```python
from build123d import *

# Parameters (mm, degrees)
SKETCH1_W            = 40
SKETCH1_H            = 40
BOSS_EXTRUDE1_DEPTH  = 650
BOSS_EXTRUDE2_START  = 550
SKETCH3_R            = 9.5
BOSS_EXTRUDE2_DEPTH  = 200
SKETCH8_R            = 150
BOSS_EXTRUDE3_DEPTH  = 10
SKETCH9_W            = 105
SKETCH9_H            = 8
SKETCH9_H_2          = 40
BOSS_EXTRUDE4_DEPTH  = 40
FILLET1_R            = 10
SKETCH10_R           = 6
CUT_EXTRUDE1_DEPTH   = 735.31209305
CUT_EXTRUDE2_DEPTH   = 767.485485838
CUT_EXTRUDE5_DEPTH   = 767.485485838
SHELL2_START         = -18
SHELL2_DEPTH         = 36
SHELL2_START_2       = 22
SHELL2_2_DEPTH       = 6
SHELL2_START_3       = 8.0000001
SHELL2_3_DEPTH       = 13.9999999
SHELL2_START_4       = -10
SHELL2_4_DEPTH       = 1.9999999
SHELL2_START_5       = -552
SHELL2_5_OUTLINE_W   = 36
SHELL2_5_OUTLINE_H   = 8
SHELL2_5_OUTLINE_H_2 = 16.0000002
SHELL2_5_DEPTH       = 1300
SHELL2_6_OUTLINE_W   = 105
SHELL2_6_OUTLINE_H   = 8
SHELL2_6_OUTLINE_H_2 = 16.0000002
SHELL2_6_DEPTH       = 36
SHELL2_START_6       = -748
SHELL2_7_OUTLINE_R   = 7.5
SHELL2_7_DEPTH       = 196
SHELL2_START_7       = 552
SHELL2_8_DEPTH       = 196
SHELL2_START_8       = -66
SHELL2_9_DEPTH       = 4
SHELL2_START_9       = 62
SHELL2_10_DEPTH      = 4
SKETCH12_R           = 12.5
CUT_EXTRUDE3_DEPTH   = 70
SKETCH13_W           = 30
SKETCH13_H           = 30
CUT_EXTRUDE4_DEPTH   = 20


with BuildPart() as part:
    # Sketch1 → Boss-Extrude1 (new, symmetric)
    with BuildSketch(Plane.XY):
        Rectangle(SKETCH1_W, SKETCH1_H)
    extrude(amount=BOSS_EXTRUDE1_DEPTH, both=True)

    # Sketch3 → Boss-Extrude2 (add)
    with BuildSketch(Plane.XY.offset(BOSS_EXTRUDE2_START)):
        with Locations(Location((0, 25, 0), (0, 0, 211.756863859))):
            Circle(SKETCH3_R)
    boss_extrude2 = extrude(amount=BOSS_EXTRUDE2_DEPTH)

    # Sketch8 → Boss-Extrude3 (add)
    with BuildSketch(Plane(origin=(0, 20, 0), x_dir=(1, 0, 0), z_dir=(0, 1, 0))):
        with Locations(Location((0, 0, 0), (0, 0, 277.662255661))):
            Circle(SKETCH8_R)
    extrude(amount=BOSS_EXTRUDE3_DEPTH)

    # Sketch9 → Boss-Extrude4 (add)
    with BuildSketch(Plane.XZ.offset(-20)):
        with Locations((72.5, -64)):
            Rectangle(SKETCH9_W, SKETCH9_H)
        with Locations((72.5, 64)):
            Rectangle(SKETCH9_W, SKETCH9_H)
        with Locations((-72.5, 0)):
            Rectangle(SKETCH9_W, SKETCH9_H_2)
    extrude(amount=BOSS_EXTRUDE4_DEPTH)

    # Fillet1
    fillet1_edges = [part.edges().sort_by_distance(p)[0] for p in [
        (125, -20, -64),
        (125, -20, 64),
    ]]
    fillet(fillet1_edges, radius=FILLET1_R)

    # Sketch10 → Cut-Extrude1 (cut, through all)
    with BuildSketch(Plane.XY.offset(68)):
        with Locations((105, 0)):
            Circle(SKETCH10_R)
    extrude(amount=-CUT_EXTRUDE1_DEPTH, mode=Mode.SUBTRACT)

    # Sketch11 → Cut-Extrude2 (cut, through all)
    with BuildSketch(Plane(origin=(0, 30, 0), x_dir=(1, 0, 0), z_dir=(0, 1, 0))):
        with BuildLine():
            Line((105, 17.5), (150, 17.5))
            Line((150, 17.5), (150, -17.5))
            Line((150, -17.5), (105, -17.5))
            ThreePointArc((105, -17.5), (87.5, 0), (105, 17.5))
        make_face()
    extrude(amount=-CUT_EXTRUDE2_DEPTH, mode=Mode.SUBTRACT)

    # Mirror1: Boss-Extrude2 across plane
    add(boss_extrude2.mirror(Plane.XY))

    # Sketch14 → Cut-Extrude5 (cut, through all)
    with BuildSketch(Plane(origin=(0, 30, 0), x_dir=(1, 0, 0), z_dir=(0, 1, 0))):
        with BuildLine():
            Line((-106.066017178, 106.066017178), (-98.994949366, 98.994949366))
            ThreePointArc((-98.994949366, 98.994949366), (-140, 0), (-98.994949366, -98.994949366))
            Line((-98.994949366, -98.994949366), (-106.066017178, -106.066017178))
            ThreePointArc((-106.066017178, -106.066017178), (-150, 0), (-106.066017178, 106.066017178))
        make_face()
    extrude(amount=-CUT_EXTRUDE5_DEPTH, mode=Mode.SUBTRACT)

    # Shell2: read off the stored shape, not the designer's step
    # Shell2 outline → Shell2 (cut)
    with BuildSketch(Plane(origin=(0, 0, 0), x_dir=(1, 0, 0), z_dir=(0, 1, 0)).offset(SHELL2_START)):
        with BuildLine():
            Line((-18, 648), (-18, 146.901327428))
            ThreePointArc((-18, 146.901327428), (0, 148), (18, 146.901327428))
            Line((18, 146.901327428), (18, 648))
            Line((18, 648), (-18, 648))
        make_face()
        with BuildLine():
            ThreePointArc((18, -146.901327428), (0, -148), (-18, -146.901327428))
            Line((-18, -146.901327428), (-18, -650))
            Line((-18, -650), (18, -650))
            Line((18, -650), (18, -146.901327428))
        make_face()
    extrude(amount=SHELL2_DEPTH, mode=Mode.SUBTRACT)

    # Shell2 2 outline → Shell2 2 (cut)
    with BuildSketch(Plane(origin=(0, 0, 0), x_dir=(1, 0, 0), z_dir=(0, 1, 0)).offset(SHELL2_START_2)):
        with BuildLine():
            Line((-103.22803412, 106.056461245), (-96.156273779, 98.984700904))
            ThreePointArc((-96.156273779, 98.984700904), (-138, 0), (-96.156273779, -98.984700904))
            Line((-96.156273779, -98.984700904), (-103.22803412, -106.056461245))
            ThreePointArc((-103.22803412, -106.056461245), (48.432118419, -139.85109905), (146.709747461, -19.5))
            Line((146.709747461, -19.5), (105, -19.5))
            ThreePointArc((105, -19.5), (85.5, 0), (105, 19.5))
            Line((105, 19.5), (146.709747461, 19.5))
            ThreePointArc((146.709747461, 19.5), (48.432118419, 139.85109905), (-103.22803412, 106.056461245))
        make_face()
    extrude(amount=SHELL2_2_DEPTH, mode=Mode.SUBTRACT)

    # Shell2 3 outline → Shell2 3 (cut)
    with BuildSketch(Plane(origin=(0, 0, 0), x_dir=(1, 0, 0), z_dir=(0, 1, 0)).offset(SHELL2_START_3)):
        with BuildLine():
            ThreePointArc((18, 146.901327428), (0, 148), (-18, 146.901327428))
            Line((-18, 146.901327428), (-18, 18))
            Line((-18, 18), (-123, 18))
            Line((-123, 18), (-123, -18))
            Line((-123, -18), (-18, -18))
            Line((-18, -18), (-18, -146.901327428))
            ThreePointArc((-18, -146.901327428), (0, -148), (18, -146.901327428))
            Line((18, -146.901327428), (18, -66))
            Line((18, -66), (123, -66))
            Line((123, -66), (123, -62))
            Line((123, -62), (18, -62))
            Line((18, -62), (18, 62))
            Line((18, 62), (123, 62))
            Line((123, 62), (123, 66))
            Line((123, 66), (18, 66))
            Line((18, 66), (18, 146.901327428))
        make_face()
    extrude(amount=SHELL2_3_DEPTH, mode=Mode.SUBTRACT)

    # Shell2 4 outline → Shell2 4 (cut)
    with BuildSketch(Plane(origin=(0, 0, 0), x_dir=(1, 0, 0), z_dir=(0, 1, 0)).offset(SHELL2_START_4)):
        with BuildLine():
            ThreePointArc((18, 146.901327428), (0, 148), (-18, 146.901327428))
            Line((-18, 146.901327428), (-18, 18))
            Line((-18, 18), (-123, 18))
            Line((-123, 18), (-123, -18))
            Line((-123, -18), (-18, -18))
            Line((-18, -18), (-18, -146.901327428))
            ThreePointArc((-18, -146.901327428), (0, -148), (18, -146.901327428))
            Line((18, -146.901327428), (18, -66))
            Line((18, -66), (123, -66))
            Line((123, -66), (123, -62))
            Line((123, -62), (18, -62))
            Line((18, -62), (18, 62))
            Line((18, 62), (123, 62))
            Line((123, 62), (123, 66))
            Line((123, 66), (18, 66))
            Line((18, 66), (18, 146.901327428))
        make_face()
    extrude(amount=SHELL2_4_DEPTH, mode=Mode.SUBTRACT)

    # Shell2 5 outline → Shell2 5 (cut)
    with BuildSketch(Plane.XY.offset(SHELL2_START_5)):
        with Locations((0, -14)):
            Rectangle(SHELL2_5_OUTLINE_W, SHELL2_5_OUTLINE_H)
        Rectangle(SHELL2_5_OUTLINE_W, SHELL2_5_OUTLINE_H_2)
        with BuildLine():
            Line((2.692582404, 18), (-2.692582404, 18))
            ThreePointArc((-2.692582404, 18), (0, 17.5), (2.692582404, 18))
        make_face()
    extrude(amount=SHELL2_5_DEPTH, mode=Mode.SUBTRACT)

    # Shell2 6 outline → Shell2 6 (cut)
    with BuildSketch(Plane.XY.offset(SHELL2_START)):
        with Locations((-70.5, -14)):
            Rectangle(SHELL2_6_OUTLINE_W, SHELL2_6_OUTLINE_H)
        with Locations((-70.5, 0)):
            Rectangle(SHELL2_6_OUTLINE_W, SHELL2_6_OUTLINE_H_2)
    extrude(amount=SHELL2_6_DEPTH, mode=Mode.SUBTRACT)

    # Shell2 7 outline → Shell2 7 (cut)
    with BuildSketch(Plane.XY.offset(SHELL2_START_6)):
        with Locations((0, 25)):
            Circle(SHELL2_7_OUTLINE_R)
    extrude(amount=SHELL2_7_DEPTH, mode=Mode.SUBTRACT)

    # Shell2 8 outline → Shell2 8 (cut)
    with BuildSketch(Plane.XY.offset(SHELL2_START_7)):
        with BuildLine():
            ThreePointArc((2.692582404, 18), (0, 32.5), (-2.692582404, 18))
            Line((-2.692582404, 18), (2.692582404, 18))
        make_face()
    extrude(amount=SHELL2_8_DEPTH, mode=Mode.SUBTRACT)

    # Shell2 9 outline → Shell2 9 (cut)
    with BuildSketch(Plane.XY.offset(SHELL2_START_8)):
        with BuildLine():
            Line((18, -10), (18, -18))
            Line((18, -18), (115, -18))
            ThreePointArc((115, -18), (120.656854249, -15.656854249), (123, -10))
            Line((123, -10), (18, -10))
        make_face()
        with BuildLine():
            Line((18, 8.0000001), (18, -8.0000001))
            Line((18, -8.0000001), (105, -8))
            ThreePointArc((105, -8), (97, 0), (105, 8))
            Line((105, 8), (18, 8.0000001))
        make_face()
        with BuildLine():
            ThreePointArc((105, 8), (113, 0), (105, -8))
            Line((105, -8), (123, -8.0000001))
            Line((123, -8.0000001), (123, 8.0000001))
            Line((123, 8.0000001), (105, 8))
        make_face()
    extrude(amount=SHELL2_9_DEPTH, mode=Mode.SUBTRACT)

    # Shell2 10 outline → Shell2 10 (cut)
    with BuildSketch(Plane.XY.offset(SHELL2_START_9)):
        with BuildLine():
            Line((18, -10), (18, -18))
            Line((18, -18), (115, -18))
            ThreePointArc((115, -18), (120.656854249, -15.656854249), (123, -10))
            Line((123, -10), (18, -10))
        make_face()
        with BuildLine():
            Line((18, 8.0000001), (18, -8.0000001))
            Line((18, -8.0000001), (105, -8))
            ThreePointArc((105, -8), (97, 0), (105, 8))
            Line((105, 8), (18, 8.0000001))
        make_face()
        with BuildLine():
            ThreePointArc((105, 8), (113, 0), (105, -8))
            Line((105, -8), (123, -8.0000001))
            Line((123, -8.0000001), (123, 8.0000001))
            Line((123, 8.0000001), (105, 8))
        make_face()
    extrude(amount=SHELL2_10_DEPTH, mode=Mode.SUBTRACT)

    # Sketch12 → Cut-Extrude3 (cut)
    with BuildSketch(Plane(origin=(0, 30, 0), x_dir=(1, 0, 0), z_dir=(0, 1, 0))):
        with Locations(Location((0, 0, 0), (0, 0, 180))):
            Circle(SKETCH12_R)
    extrude(amount=-CUT_EXTRUDE3_DEPTH, mode=Mode.SUBTRACT)

    # Sketch13 → Cut-Extrude4 (cut)
    with BuildSketch(Plane.XZ.offset(20)):
        Rectangle(SKETCH13_W, SKETCH13_H)
    extrude(amount=-CUT_EXTRUDE4_DEPTH, mode=Mode.SUBTRACT)


solid = part.part
```
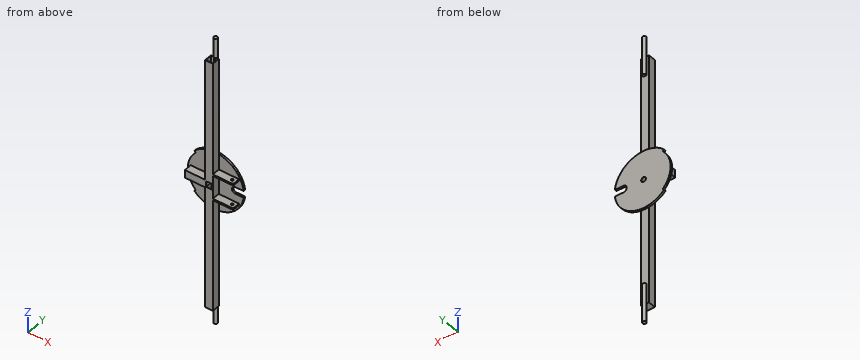
Read the model definition and answer for the solid it produces. Units are mm, in the model's axes. Coordinates: 2 decimals unless noted, no trailing zeros. Write each loop counter-clockwise with the first axis right and the second up, starting at its lowest first coordinate (ties: lowest second). Pieces come first, ordered by that corner, then holes. Notation, with made-up numbers: (-19, 32.5) -> (-10, 32.5) arc R32 ccw to (-10, 71.5) -> close; hole circle Ø6 at (6.5, -8). An arc over 180 degrees is marked (long way). Answer as a JSON object with one key per item and string values.
Q1. Consider line 1 (Z direction, x = 84, y = -8); line 2 (X direction, y = 12, z = -474); line 3 (Y direction, x = -16.5, z = 55). Determine where each line is inside the solid, lowest interval first. Write a range as [from, to].
The answers:
{"line 1": "z = [-68, -66], [-62, -60], [60, 62], [66, 68]", "line 2": "x = [-20, -18], [18, 20]", "line 3": "y = [-20, -18], [28, 30]"}
Q2. Flat-ended cylindrical pins translate along their axes: pin 1 Ø11 at (x, y) = (136.5, 27) entering from -Z; pin 2 Ø20 at (x, y) = (77, 5) entering from -Z; pin 3 Ø5 at (x, y) = (131.5, 27) entering from +Z. Find the tip coordinate at first contact, or state that the pin passes through.
The answers:
{"pin 1": "stops at z = -73.07", "pin 2": "stops at z = -68", "pin 3": "stops at z = 76.54"}
Q3. The part is cut by section B-B on z = 0. Give the vertices of the cut face in (x, y), then the cut area to 3 significant figures.
The answers:
{"outline": "(-140, 20) -> (-125, 20) -> (-125, -20) -> (-15, -20) -> (-15, -18) -> (-123, -18) -> (-123, 22) -> (-138, 22) -> (-138, 28) -> (-12.5, 28) -> (-12.5, 30) -> (-140, 30) -> close; (12.5, 28) -> (85.5, 28) -> (85.5, 22) -> (18, 22) -> (18, -18) -> (15, -18) -> (15, -20) -> (20, -20) -> (20, 20) -> (87.5, 20) -> (87.5, 30) -> (12.5, 30) -> close", "area": "984 mm2"}
Q4. The part is cut by section A-A on z = 317. Give the vertices of the cut face in (x, y).
The answers:
{"outline": "(-20, -20) -> (20, -20) -> (20, 20) -> (-20, 20) -> close; hole (-18, -18) -> (18, -18) -> (18, 18) -> (-18, 18) -> close"}
Q5. The part is cut by section C-C on x = 47. Give the vertices of the cut face in (y, z).
The answers:
{"outline": "(-20, -68) -> (20, -68) -> (20, -142.45) -> (30, -142.45) -> (30, 142.45) -> (20, 142.45) -> (20, 68) -> (-20, 68) -> (-20, 60) -> (20, 60) -> (20, -60) -> (-20, -60) -> close; hole (-18, -66) -> (22, -66) -> (22, -140.34) -> (28, -140.34) -> (28, 140.34) -> (22, 140.34) -> (22, 66) -> (-18, 66) -> (-18, 62) -> (22, 62) -> (22, -62) -> (-18, -62) -> close"}
